Geometry check sheet. Reference: the model listing, model coordinates, mm. A direction names the side the tool comes from. Give positions to 0.01 mm unless a question says otherwise; leave off trailing zeros. Order: outer loops, then holes, each group sorted by start corner. A loop starts at its lowest first (then second) coordinate and runs counter-clockwise, first axis right, second up.
Autodesk Inventor part; units mm, degrees
ref_plane "Work Plane1" through (1.525, 0, 0) normal (0, 0, 1) x (1, 0, 0)
ref_plane "YZ Plane" through (0, 0, 0) normal (1, 0, 0) x (0, 1, 0)
ref_plane "XZ Plane" through (0, 0, 0) normal (0, 1, 0) x (-1, 0, 0)
sketch "Sketch1" plane through (0, 0, 0) normal (0, 0, 1) x (1, 0, 0)
  line L0 (0, 14.095) -> (0, 10)
  line L1 (34, 10) -> (80, 10)
  line L2 (80, 10) -> (80, 0)
  line L3 (80, 0) -> (-0.8001, 0)
  line L4 (-16.9601, 0) -> (96.16, 0)
  line L5 (-0.8001, 0) -> (-0.8001, 14.095)
  line L6 (-0.8001, 14.095) -> (0, 14.095)
  line L7 (34, 10) -> (32.773, 10)
  line L8 (32.773, 10) -> (0, 10)
  line L9 (0, -2.819) -> (0, 16.914)
  dimension "d0" = 80
  dimension "d1" = 46
  dimension "d2" = 20
  dimension "d9" = 0.8001
  dimension "d10" = 28.19
  dimension "d13" = 1.227
  dimension "d14" = 20
revolve "Body" add sketch "Sketch1" angle 360 about axis through (80, 0, 0) along (-1, 0, 0)
sketch "Sketch2" plane through (-0.8001, 0, 0) normal (-1, 0, 0) x (0, 0, 1)
  line L0 (0, 17.3205) -> (15, 8.6603)
  line L1 (15, 8.6603) -> (15, -8.6603)
  line L2 (15, -8.6603) -> (0, -17.3205)
  line L3 (0, -17.3205) -> (-15, -8.6603)
  line L4 (-15, -8.6603) -> (-15, 8.6603)
  line L5 (-15, 8.6603) -> (0, 17.3205)
  point P0 (0, 0)
  point P1 (0, 0)
  dimension "d11" = 30
extrude "Head" add sketch "Sketch2" along normal blind 11.7
sketch "Sketch4" plane through (0, 0, 0) normal (0, 0, 1) x (1, 0, 0)
  line L0 (-12.5001, 15) -> (-12.5001, 17.3205)
  line L1 (-12.5001, 17.3205) -> (-11.1604, 17.3205)
  line L2 (-11.1604, 17.3205) -> (-12.5001, 15)
  line L3 (-14.8401, 0) -> (1.5399, 0)
  line L4 (-0.8001, 17.3205) -> (-12.5001, 17.3205)
  line L5 (-12.5001, 8.6603) -> (-12.5001, 17.3205)
  dimension "d5" = 30
  dimension "d19" = 30
revolve "Chamfer1" cut sketch "Sketch4" angle 360 about axis through (-10, 0, 0) along (1, 0, 0)
thread "Thread"
chamfer "Chamfer2" distance 1.2269 distance2 1.227 1 edges at (80, -10, 0) measured on face at (80, -2.8768, 3.7595)
ref_plane "Work Plane1" through (1.525, 0, 0) normal (0, 0, 1) x (1, 0, 0)
equation "\"d0\" = NLG"
equation "\"d1\" = GEL"
equation "\"d2\" = GD"
equation "\"d10\" = SD2"
equation "\"d14\" = BDM"
equation "\"d11\" = SW"
equation "\"d3\" = KOH - SD"
equation "\"d5\" = ANG1"
equation "\"d19\" = SW0"
equation "\"d15\" = GEL"
equation "\"d6\" = -0.5 * SPD + 0.5 * GD"
equation "\"NLG\" = 80"
equation "\"GD\" = NND"
equation "\"BDM\" = NND"
equation "\"KOH\" = 12.5"
equation "\"GEL\" = 46"
equation "\"SW\" = 30"
equation "\"SW0\" = SW"
equation "\"SPD\" = NND - 1.2269 * PTC"
equation "\"SD2\" = 28.19"
equation "\"SD\" = 0.8"
equation "\"ANG1\" = 30deg"
equation "\"GAL\" = 0.61345 * PTC"
equation "\"GUL\" = 0.61345 * PTC"
equation "\"RR\" = 0.8"
equation "\"GD1\" = THREADDIA - 1.2269 * PTC"
equation "\"SDH\" = SD2"
equation "\"TOA\" = 30deg"
equation "\"PTC\" = 2"
equation "\"E0\" = 1.155 * SW"
properties part number "ISO 8765 - M20 x 2 x 80" material "Stainless Steel, 440C"
Item 1: Gauge pin test, flat ends, axial feed: pin 1 (8 mm diameter, centred on x = 70.5, z = -4.5, fed in from +Y); pin 2 (8 mm diameter, centred on x = 17.5, y = -9.5, fed in from +Z); pin 3 (8 mm diameter, centred on x = 60, z = 4.5, fed in from -Y). Record the tip position at first contact, or that the pin passes through.
Reported:
pin 1: stops at y = 9.99
pin 2: stops at z = 8.35
pin 3: stops at y = -9.99
Item 2: Sectioned sample at A-A (x = 54.5). Enter the section's corners in (y, z), and give its area (3 significant figures).
Reported:
outline: circle Ø20 at (0, 0)
area: 314 mm2
Item 3: Scan lines: L1, parallel to Y at x = 6.5, z = 0; L2, parallel to X at y = 8, z = -9; L3, parallel to X at y = -10.5, z = -9.5. Record each from-to range of solid material in increasing order.
Reported:
L1: y = -10 to 10
L2: x = -12.5 to 0
L3: x = -12.5 to -0.8
Item 4: Set-up check for faces 1 (the flat face through (-0.8, -14, -3)), 2 (the flat face through (-6.57, 13.05, 7.4)): record each of +Z, -Z, +X, -X, +Y, -Y from which the full face is reachable in a straight line by a thin tool's end or side.
Reported:
face 1: +X
face 2: +Z, +X, -X, +Y
